Source: three-view drawing plus pictorial views. Frame: mm from the lowest corner of the part. A direction names the side the tool comes from. Round coordinates to 2 decimals unless told otherwise and drop trailing zeros. Write each loop counter-clockwise with the first axis right and the second up, starting at its lowest first coordinate (ties: lowest second). Pieces come first, ordered by that corner, then holes. Notation, with made-up numbers: M 55.5,-2.75 L 106.5,-2.75 A10 ccw 106.5,6.25 Z; hole C -32.5,-38.75 d7. An arc over 180 degrees is marked long. Answer in a Markdown table with one row per item.
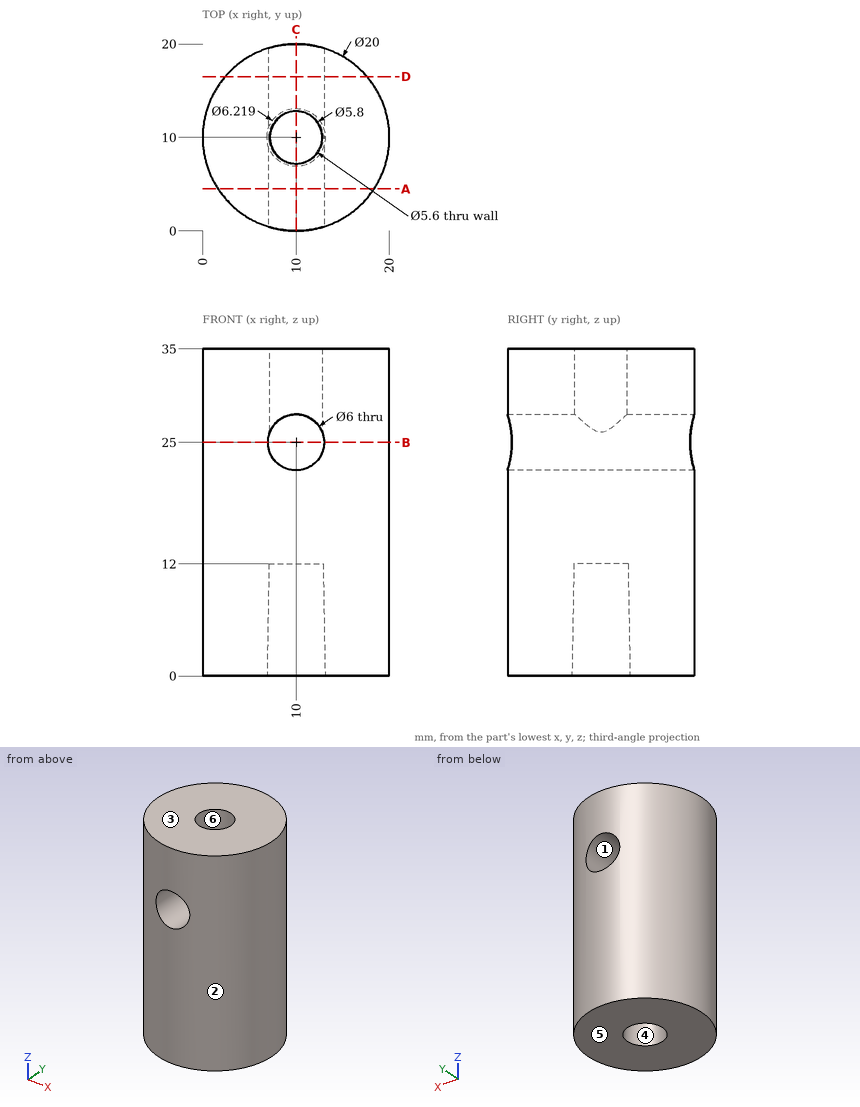
Q1. Access query for the marked faces 5 and 6. Directions: +Z, -Z, +X, -X, +Y, -Y. A direction counts if a zero-diameter tool reaches every point of the face in a straight line with its end or side. Return the directions, or none.
Solutions:
| item | result |
|---|---|
| face 5 | -Z, +X, -X, +Y, -Y |
| face 6 | +Z |
Q2. Pull-direction query (X, two-part tool) for the marked faces 1, 2, 3 and 4; classes: pulls with the +X half, pulls with the -X half, needs draft (parallel to the pull), parting line crosses it, or undercut.
Solutions:
| item | result |
|---|---|
| face 1 | undercut |
| face 2 | parting line crosses it |
| face 3 | needs draft |
| face 4 | undercut |
Q3. Section A-A (y = 4.5). Return loops of the section in (x, z).
Solutions:
| item | result |
|---|---|
| outline | M 1.65,0 L 18.35,0 L 18.35,35 L 1.65,35 Z; hole C 10,25 d6 |
Q4. Section D-D (y = 16.5). Return loops of the section in (x, z).
Solutions:
| item | result |
|---|---|
| outline | M 2.4,0 L 17.6,0 L 17.6,35 L 2.4,35 Z; hole C 10,25 d6 |
Q5. Section C-C (x = 10). State how many separate pieces and enclosed holes the cut face has, and give its area (3 significant figures).
Solutions:
| item | result |
|---|---|
| separate pieces | 3 |
| enclosed holes | 0 |
| area | 469 mm2 |
Q6. Material intervals for probe 1 along Y at (x, z) = (10, 29.75); probe 2 along X at (y, z) = (12.75, 2.5) (1 decimal); probe 3 along X at (y, z) = (6, 27.5) (1 decimal), sorted ascending.
Solutions:
| item | result |
|---|---|
| probe 1 | y = 0 to 7.2, 12.8 to 20 |
| probe 2 | x = 0.4 to 8.6, 11.4 to 19.6 |
| probe 3 | x = 0.8 to 8.3, 11.7 to 19.2 |
Q7. Section B-B (z = 25). Return loops of the section in (x, y).
Solutions:
| item | result |
|---|---|
| outline | M 7,0.46 L 7,19.54 A10 ccw Z; M 13,0.46 A10 ccw 13,19.54 Z |
Q8. Contact query for flat-ended pins moving along their axis: pin 1 Ø12 at (x, z) = (16.5, 4) entering from +Y; pin 2 Ø8 at (x, z) = (12, 15) entering from -Y; pin 3 Ø4 at (x, z) = (15, 27.5) entering from +Y; pin 4 Ø5 at (x, z) = (10, 25) entering from +Y. Output: stop coordinate, or through.
Solutions:
| item | result |
|---|---|
| pin 1 | stops at y = 19.99 |
| pin 2 | stops at y = 0 |
| pin 3 | stops at y = 19.54 |
| pin 4 | passes through |
